Geometry: final body of the model. Coordinates: model frame, mm. Give positions to 0.01 mm unless a question says otherwise; leave off trailing zeros. Loops run counter-clockwise (first coordinate to the right, second up) from the corner with the lowest first, then second, coordinate; pieces in that order, holes last. Notation, with made-up numbers: (57.5, 80) - (111.5, 80) arc R6 cw to (111.5, 90) - close; hole circle Ø5 at (27.25, 32). An arc over 180 degrees is marked (long way). Answer in a Markdown table with one row per item.
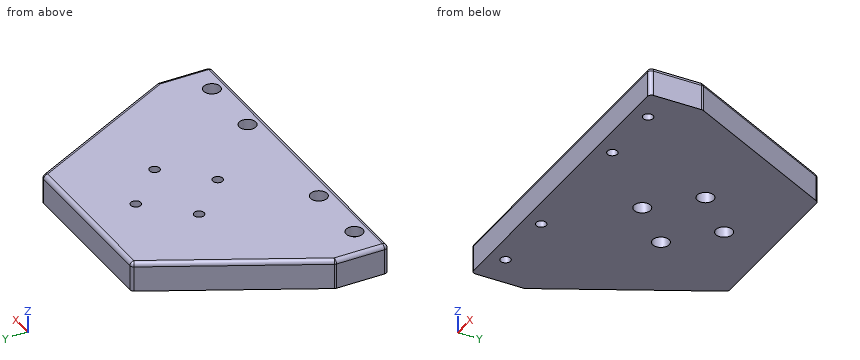
from build123d import *

# Parameters (mm, degrees)
F1_DEPTH       = 18
F2_D           = 6.2
F2_CBORE_D     = 10.2
F2_CBORE_DEPTH = 7
F4_D           = 6.2
F4_CBORE_D     = 10.2
F4_CBORE_DEPTH = 6.5
F5_R           = 2.5


with BuildPart() as f1:
    # F0 (on Top) → F1 (new body)
    with BuildSketch(Plane.XY):
        Polygon((-80, 0), (0, 0), (100, 0), (100, 32.5), (50, 130), (0, 130), (-50, 130), (-100, 32.5), (-100, 0), align=None)
    extrude(amount=F1_DEPTH)

    # F2 (through all)
    with Locations(Plane(origin=(0, 0, 0), x_dir=(1, 0, 0), z_dir=(0, 0, -1))):
        with Locations((0, -100), (25, -75), (0, -50), (-25, -75)):
            CounterBoreHole(F2_D / 2, F2_CBORE_D / 2, F2_CBORE_DEPTH)

    # F4 (through all)
    with Locations(Plane.XY.offset(18)):
        with Locations((-80, 10), (-40, 10), (40, 10), (80, 10)):
            CounterBoreHole(F4_D / 2, F4_CBORE_D / 2, F4_CBORE_DEPTH)

    # F5
    f5_edges = [f1.edges().sort_by_distance(p)[0] for p in [
        (-100, 32.5, 9),
        (-100, 16.25, 18),
        (0, 0, 18),
        (100, 16.25, 18),
        (-75, 81.25, 18),
        (75, 81.25, 18),
        (50, 130, 9),
        (-50, 130, 9),
        (100, 0, 9),
        (-100, 0, 9),
        (100, 32.5, 9),
        (0, 130, 18),
    ]]
    fillet(f5_edges, radius=F5_R)


solid = f1.part
Q1. Material intervals for line 1 along Y through (x, z) = (0, 2.5); line 2 along Y through (x, z) = (4, 3.25); line 3 along Y through (x, z) = (-25, 13), sorted ascending.
Check values:
| item | result |
|---|---|
| line 1 | 0 to 44.9, 55.1 to 94.9, 105.1 to 130 |
| line 2 | 0 to 46.84, 53.16 to 96.84, 103.16 to 130 |
| line 3 | 0 to 71.9, 78.1 to 130 |
Q2. Cut plane C-C (y = 10). Give the number of separate pieces and of enclosed holes in the cut face, and give its area (3 significant figures).
Check values:
| item | result |
|---|---|
| separate pieces | 5 |
| enclosed holes | 0 |
| area | 3,050 mm² |
Q3. Cut plane B-B (x = -40). Output: boundary loops of the cut face in (y, z).
Check values:
| item | result |
|---|---|
| outline | (0, 0) - (6.9, 0) - (6.9, 11.5) - (4.9, 11.5) - (4.9, 18) - (2.5, 18) arc R2.5 ccw to (0, 15.5) - close; (13.1, 0) - (130, 0) - (130, 15.5) arc R2.5 ccw to (127.5, 18) - (15.1, 18) - (15.1, 11.5) - (13.1, 11.5) - close |
Q4. First-contact query: pin 1 (5.5 mm diameter, centred on x = 25, y = 75, fed in from -Z); pin 2 (8 mm diameter, centred on y = 80.5, z = 9.5, fed in from +X); pin 3 (8 mm diameter, centred on x = -25, y = 75, fed in from -Z); pin 4 (3 mm diameter, centred on y = 59.5, z = 2, fed in from -X). Flat tips, straight axial feed; report the tip coordinate or a pass-through.
Check values:
| item | result |
|---|---|
| pin 1 | through |
| pin 2 | x = 77.44 |
| pin 3 | z = 7 |
| pin 4 | x = -86.92 |
Q5. Cut plane A-A (x = 25). Output: boundary loops of the cut face in (y, z), and give its area (3 significant figures).
Check values:
| item | result |
|---|---|
| outline | (0, 0) - (69.9, 0) - (69.9, 7) - (71.9, 7) - (71.9, 18) - (2.5, 18) arc R2.5 ccw to (0, 15.5) - close; (78.1, 7) - (80.1, 7) - (80.1, 0) - (130, 0) - (130, 15.5) arc R2.5 ccw to (127.5, 18) - (78.1, 18) - close |
| area | 2,200 mm² |
